Can you work these out from the drawing? Everything is in mm from the part's minimum corner. A direction names the side the tool comes from. Round coordinates to 2 decimals unless told otherwise and drop trailing zeros. Write each loop counter-clockwise with the first axis right and the second up, starting at its lowest first coordinate (ties: lowest second). Pieces come first, ordered by that corner, then holes. Notation, with made-up numbers: M -31.5,3.25 L 26.5,3.25 A25 ccw 26.5,39.25 Z; hole C 63.25,7 d6. An arc over 180 degrees is marked long. Use one line per item in the form item = value. Start each with the question number.
Q1. I want a section at C-C on y = 16. List the corners of the cut face in (x, z) for me, and give its area (3 significant figures).
Q2. I want a section at A-A on z = 5. State how many separate pieces and enclosed holes the cut face has, and give its area (3 significant figures).
Q3. I need wall thicknesses on line 1 along X through (y, z) = (6.5, 2.5) (1 decimal); line 2 along X through (y, z) = (16, 3.5); line 3 along X through (y, z) = (9.25, 7.25). Which ranges of each line are inside material? Lowest first, please. Write a range as from..to.
Q4. I'm going to push a flat-ended pin straight in: pin 1 Ø3 at (x, z) = (36.5, 5.5) entering from +Y. Where does the tip first touch, or does it pass through?
Q5. We'd pull the mould along X, two halves only. Please class the marked faces 1, 2 and 3: +X half, -X half, draft (parallel to the pull), parting line (faces both ways), or undercut.
Q6. For the marked faces 4 and 5, which set-ups out of +Z, -Z, +X, -X, +Y, -Y let a thin tool reach every point of the face, with its end or its side?
Q7. I want a section at D-D on y = 9. List the corners of the cut face in (x, z) for me, and give its area (3 significant figures).
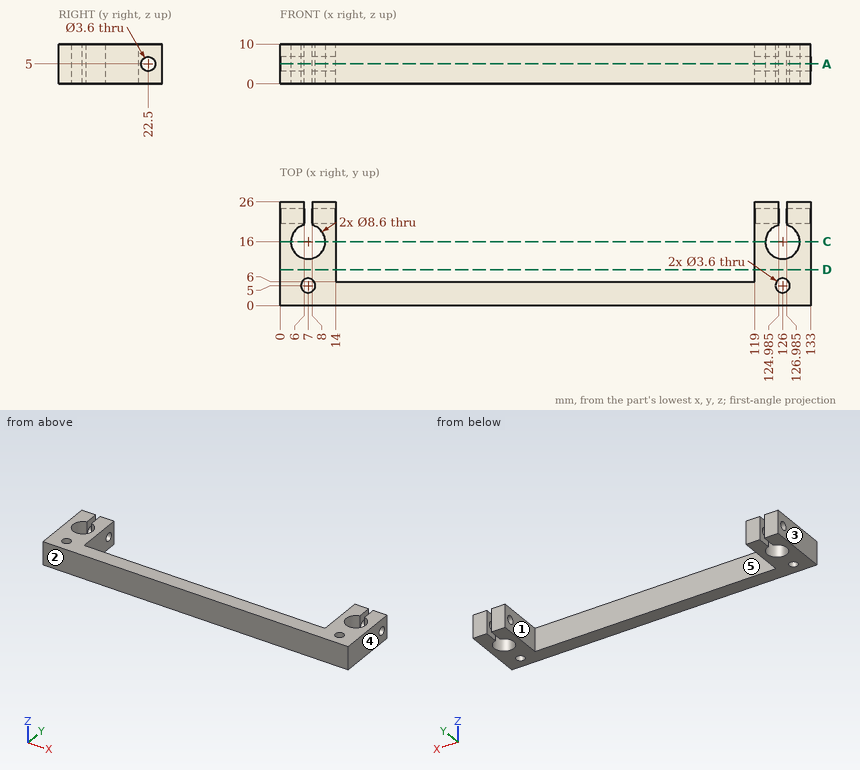
Reported:
q1.outline = M 0,0 L 2.7,0 L 2.7,10 L 0,10 Z; M 11.3,0 L 14,0 L 14,10 L 11.3,10 Z; M 119,0 L 121.7,0 L 121.7,10 L 119,10 Z; M 130.3,0 L 133,0 L 133,10 L 130.3,10 Z
q1.area = 108 mm^2
q2.separate_pieces = 5
q2.enclosed_holes = 2
q2.area = 1,110 mm^2
q3.line_1 = 0..6, 8..14, 119..125, 127..133
q3.line_2 = 0..2.7, 11.3..14, 119..121.7, 130.3..133
q3.line_3 = 0..14, 119..133
q4.pin_1 = 6
q5.face_1 = undercut
q5.face_2 = draft
q5.face_3 = -X half
q6.face_4 = +Z, -Z, +X, +Y, -Y
q6.face_5 = +Z, -Z, +Y
q7.outline = M 0,0 L 14,0 L 14,10 L 0,10 Z; M 119,0 L 133,0 L 133,10 L 119,10 Z
q7.area = 280 mm^2
